The listing builds one solid part. Answer for the finished solid, in the listing's coordinates (mm). Coordinates: 2 decimals unless noted, no trailing zeros. Order: outer loops, then holes, each group sorted by start corner. A loop starts at its lowest first (then second) coordinate and runs counter-clockwise, first axis right, second up. Notation, with made-up numbers: (20.25, -38) -> (77.25, -38) arc R15 cw to (77.25, -18) -> close; hole circle Ø1 at (-39.75, 20.25). An arc over 180 degrees is marked (long way). Put each result on its own line as item: value. Start each with the question number.
```python
from build123d import *

# Parameters (mm, degrees)
F1_DEPTH = 3
F3_DEPTH = 12.5


with BuildPart() as f1:
    # F0 (on Top) → F1 (new body)
    with BuildSketch(Plane.XY):
        with BuildLine():
            ThreePointArc((-4, -5.7445626465), (-6.204836823, -3.2403703492), (-7, 0))
            Line((-7, 0), (-7, -15))
            Line((-7, -15), (-4, -15))
            Line((-4, -15), (-4, -14))
            Line((-4, -14), (-4, -12))
            Line((-4, -12), (-4, -10))
            Line((-4, -10), (-4, -8))
            Line((-4, -8), (-4, -6))
            Line((-4, -6), (-4, -5.7445626465))
        make_face()
        with BuildLine():
            Line((-4, -2), (-4, 0))
            Line((-4, 0), (-7, 0))
            ThreePointArc((-7, 0), (-6.204836823, -3.2403703492), (-4, -5.7445626465))
            Line((-4, -5.7445626465), (-4, -4))
            Line((-4, -4), (-4, -2))
        make_face()
        with BuildLine():
            ThreePointArc((-4, 0), (0, 4), (4, 0))
            Line((4, 0), (7, 0))
            ThreePointArc((7, 0), (0, 7), (-7, 0))
            Line((-7, 0), (-4, 0))
        make_face()
        with BuildLine():
            Line((7, 0), (4, 0))
            Line((4, 0), (4, -2))
            Line((4, -2), (4, -4))
            Line((4, -4), (4, -5.7445626465))
            ThreePointArc((4, -5.7445626465), (6.204836823, -3.2403703492), (7, 0))
        make_face()
        with BuildLine():
            Line((7, -15), (7, 0))
            ThreePointArc((7, 0), (6.204836823, -3.2403703492), (4, -5.7445626465))
            Line((4, -5.7445626465), (4, -6))
            Line((4, -6), (4, -8))
            Line((4, -8), (4, -10))
            Line((4, -10), (4, -12))
            Line((4, -12), (4, -14))
            Line((4, -14), (4, -15))
            Line((4, -15), (7, -15))
        make_face()
        with BuildLine():
            ThreePointArc((-3.8729833462, -1), (-3.9681187851, -0.5040171699), (-4, 0))
            Line((-4, 0), (-4, -2))
            ThreePointArc((-4, -2), (-3.9681187851, -1.4959828301), (-3.8729833462, -1))
        make_face()
        with BuildLine():
            ThreePointArc((-3.8729833462, -3), (-3.9681187851, -2.5040171699), (-4, -2))
            Line((-4, -2), (-4, -4))
            ThreePointArc((-4, -4), (-3.9681187851, -3.4959828301), (-3.8729833462, -3))
        make_face()
        with BuildLine():
            Line((-4, -4), (-4, -5.7445626465))
            ThreePointArc((-4, -5.7445626465), (-3.9960908526, -5.7472826533), (-3.9921798557, -5.75))
            ThreePointArc((-3.9921798557, -5.75), (-3.9504206166, -5.3721648688), (-3.8729833462, -5))
            ThreePointArc((-3.8729833462, -5), (-3.9681187851, -4.5040171699), (-4, -4))
        make_face()
        with BuildLine():
            ThreePointArc((-3.8729833462, -7), (-3.9681187851, -6.5040171699), (-4, -6))
            Line((-4, -6), (-4, -8))
            ThreePointArc((-4, -8), (-3.9681187851, -7.4959828301), (-3.8729833462, -7))
        make_face()
        with BuildLine():
            ThreePointArc((-3.8729833462, -9), (-3.9681187851, -8.5040171699), (-4, -8))
            Line((-4, -8), (-4, -10))
            ThreePointArc((-4, -10), (-3.9681187851, -9.4959828301), (-3.8729833462, -9))
        make_face()
        with BuildLine():
            ThreePointArc((-3.8729833462, -11), (-3.9681187851, -10.5040171699), (-4, -10))
            Line((-4, -10), (-4, -12))
            ThreePointArc((-4, -12), (-3.9681187851, -11.4959828301), (-3.8729833462, -11))
        make_face()
        with BuildLine():
            Line((-4, -12), (-4, -14))
            ThreePointArc((-4, -14), (-3.9681187851, -13.4959828301), (-3.8729833462, -13))
            ThreePointArc((-3.8729833462, -13), (-3.9681187851, -12.5040171699), (-4, -12))
        make_face()
        with BuildLine():
            ThreePointArc((3.8729833462, -13), (3.9681187851, -13.4959828301), (4, -14))
            Line((4, -14), (4, -12))
            ThreePointArc((4, -12), (3.9681187851, -12.5040171699), (3.8729833462, -13))
        make_face()
        with BuildLine():
            Line((4, -12), (4, -10))
            ThreePointArc((4, -10), (3.9681187851, -10.5040171699), (3.8729833462, -11))
            ThreePointArc((3.8729833462, -11), (3.9681187851, -11.4959828301), (4, -12))
        make_face()
        with BuildLine():
            Line((4, -10), (4, -8))
            ThreePointArc((4, -8), (3.9681187851, -8.5040171699), (3.8729833462, -9))
            ThreePointArc((3.8729833462, -9), (3.9681187851, -9.4959828301), (4, -10))
        make_face()
        with BuildLine():
            Line((4, -8), (4, -6))
            ThreePointArc((4, -6), (3.9681187851, -6.5040171699), (3.8729833462, -7))
            ThreePointArc((3.8729833462, -7), (3.9681187851, -7.4959828301), (4, -8))
        make_face()
        with BuildLine():
            ThreePointArc((3.9921798557, -5.75), (3.9960908526, -5.7472826533), (4, -5.7445626465))
            Line((4, -5.7445626465), (4, -4))
            ThreePointArc((4, -4), (3.9681187851, -4.5040171699), (3.8729833462, -5))
            ThreePointArc((3.8729833462, -5), (3.9504206166, -5.3721648688), (3.9921798557, -5.75))
        make_face()
        with BuildLine():
            Line((4, -4), (4, -2))
            ThreePointArc((4, -2), (3.9681187851, -2.5040171699), (3.8729833462, -3))
            ThreePointArc((3.8729833462, -3), (3.9681187851, -3.4959828301), (4, -4))
        make_face()
        with BuildLine():
            Line((4, -2), (4, 0))
            ThreePointArc((4, 0), (3.9681187851, -0.5040171699), (3.8729833462, -1))
            ThreePointArc((3.8729833462, -1), (3.9681187851, -1.4959828301), (4, -2))
        make_face()
    extrude(amount=F1_DEPTH)

    # F2 (on Right) → F3 (cut, symmetric)
    with BuildSketch(Plane.YZ):
        Polygon((7, 3), (0, 3), (-15, 3), (-15, 0), align=None)
    extrude(amount=F3_DEPTH, both=True, mode=Mode.SUBTRACT)


solid = f1.part
```
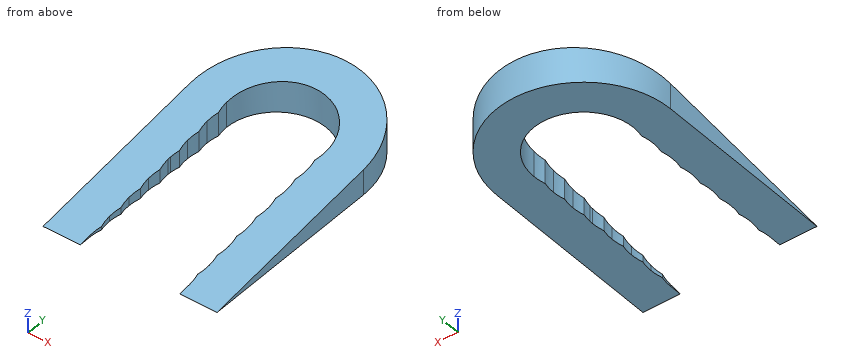
(1) The part is cut by section D-D on y = 5. Determine the outline of the cut face in (x, z).
(2) The part is cut by section B-B on y = -9.5. Determine the outline of the cut face in (x, z).
(3) Find the intervals of material crossed by L1, parallel to X at y = -10, z = 0.4; L2, parallel to X at y = -5, z = 1.3; L3, parallel to Z at x = 5.25, y = -3.75, in increasing order.
(4) Each of these flat-tipped pins is pushed along its axis until it touches: P1, Ø1, axis at y = 2, z = 2.5, coming from the -X side; P2, Ø4, axis at x = -0.5, y = -4, coming from the +Z side. Where does it stop, or does it pass through?
(5) The part is cut by section A-A on y = -12.25. Determine the outline of the cut face in (x, z) (3 decimals).
(6) The part is cut by section C-C on x = 2. Determine the outline of the cut face in (y, z), plus the area to 3 significant figures.
Worked out:
1. outline: (-4.9, 0) -> (4.9, 0) -> (4.9, 2.73) -> (-4.9, 2.73) -> close
2. outline: (-7, 0) -> (-3.97, 0) -> (-3.97, 0.75) -> (-7, 0.75) -> close; (3.97, 0) -> (7, 0) -> (7, 0.75) -> (3.97, 0.75) -> close
3. L1: -7 to -4, 4 to 7
3. L2: -7 to -3.87, 3.87 to 7
3. L3: 0 to 1.53
4. P1: x = -6.82
4. P2: through
5. outline: (-7, 0) -> (-3.992, 0) -> (-3.992, 0.375) -> (-7, 0.375) -> close; (3.992, 0) -> (7, 0) -> (7, 0.375) -> (3.992, 0.375) -> close
6. outline: (3.46, 0) -> (6.71, 0) -> (6.71, 2.96) -> (3.46, 2.52) -> close
6. area: 8.89 mm2
